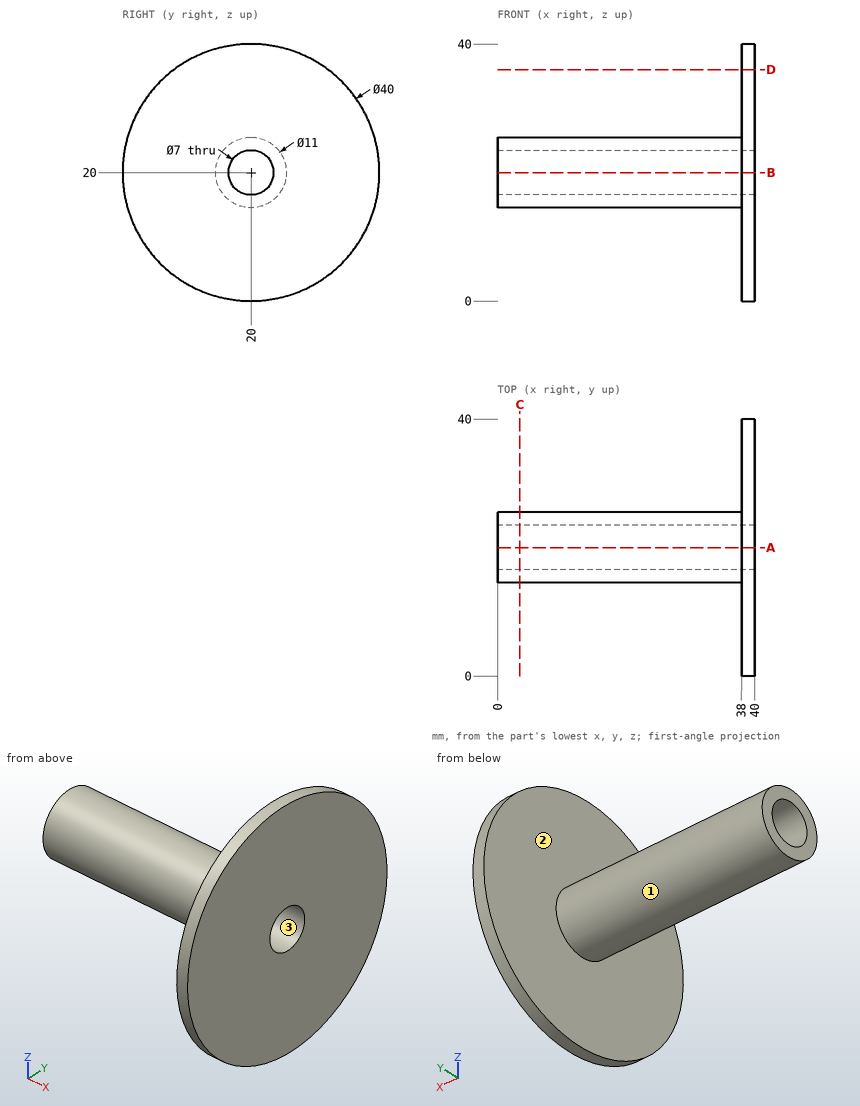
Can you work these out from the drawing? Everything is in mm from the part's minimum corner. Give positions to 0.01 mm unless a question says otherwise; leave off trailing zeros. Write each loop counter-clockwise with the first axis right and the second up, starting at its lowest first coordinate (ties: lowest second). Pieces come first, ordered by that corner, then holes. Notation, with made-up numbers: M 10,7.5 L 57,7.5 A28 cw 57,39.5 Z; hole C 60.5,12.5 d2. An arc over 180 degrees is marked long. Answer in a Markdown table with one row per item. Add a question column.
Item 1: Please list where these lines run through material, in increasing order: L1, parallel to Y at x = 26.5, z = 20; L2, parallel to X at y = 12, z = 31; L3, parallel to Y at x = 19.5, z = 25.
Item 2: Imagine slicing it at D-D, the plane z = 36. Write out the boundary of the cut face in (x, y).
Item 3: Imagine slicing it at C-C, the plane x = 3.5. Write out the boundary of the cut face in (y, z), plus the area to 3 significant figures.
Item 4: Imagine slicing it at A-A, the plane y = 20. Write out the boundary of the cut face in (x, z), plus the area to 3 significant figures.
Item 5: We'd pull the mould along Z, two halves only. Please class the marked faces 1, 2 and 3: released by +Z, released by -Z, zero draft, split by the parting line, or undercut.
Item 6: For pin 1 Ø1.5 at (y, z) = (30.5, 25.5) entering from -X; pin 2 Ø3 at (x, y) = (34, 20) entering from +Z; pin 3 Ø5 at (x, y) = (13, 14) entering from +Z, each with a flat end and sliding along its axis, tell me the tip position at first contact or that it passes through.
Evaluation:
| question | item | result |
|---|---|---|
| 1 | L1 | y = 14.5 to 16.5, 23.5 to 25.5 |
| 1 | L2 | x = 38 to 40 |
| 1 | L3 | y = 17.71 to 22.29 |
| 2 | outline | M 38,8 L 40,8 L 40,32 L 38,32 Z |
| 3 | outline | C 20,20 d11; hole C 20,20 d7 |
| 3 | area | 56.5 mm² |
| 4 | outline | M 0,14.5 L 38,14.5 L 38,0 L 40,0 L 40,16.5 L 0,16.5 Z; M 0,23.5 L 40,23.5 L 40,40 L 38,40 L 38,25.5 L 0,25.5 Z |
| 4 | area | 218 mm² |
| 5 | face 1 | split by the parting line |
| 5 | face 2 | zero draft |
| 5 | face 3 | undercut |
| 6 | pin 1 | stops at x = 38 |
| 6 | pin 2 | stops at z = 25.5 |
| 6 | pin 3 | stops at z = 24.24 |
